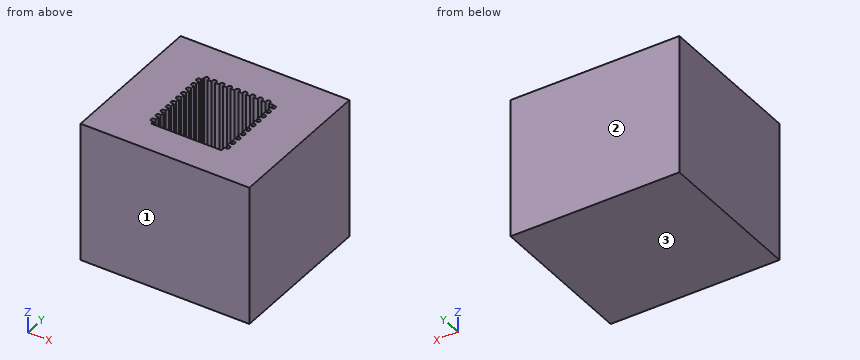
```python
from build123d import *

# Parameters (mm, degrees)
SKETCH1_W           = 504
SKETCH1_H           = 454
BOSS_EXTRUDE1_DEPTH = 416
SKETCH2_W           = 260
SKETCH2_H           = 260
CUT_EXTRUDE1_DEPTH  = 260
BOSS_EXTRUDE2_DEPTH = 260
SKETCH6_R           = 6.5
CUT_EXTRUDE2_DEPTH  = 260
LPATTERN3_COUNT     = 10
LPATTERN3_PITCH     = 23
SKETCH7_R           = 6.5
CUT_EXTRUDE3_DEPTH  = 260
LPATTERN4_COUNT     = 10
LPATTERN4_PITCH     = 23
SKETCH8_R           = 6.5
CUT_EXTRUDE4_DEPTH  = 260
LPATTERN5_COUNT     = 9
LPATTERN5_PITCH     = 23


with BuildPart() as part:
    # Sketch1 → Boss-Extrude1 (new body)
    with BuildSketch(Plane.XY):
        Rectangle(SKETCH1_W, SKETCH1_H)
    extrude(amount=-BOSS_EXTRUDE1_DEPTH)

    # Sketch2 → Cut-Extrude1 (cut)
    with BuildSketch(Plane.XY):
        Rectangle(SKETCH2_W, SKETCH2_H)
    extrude(amount=-CUT_EXTRUDE1_DEPTH, mode=Mode.SUBTRACT)

    # Sketch5 → Boss-Extrude2 (add)
    with BuildSketch(Plane.XY):
        Polygon((-105, 130), (-130, 130), (-130, 105), (-130, -130), (-105, -130), (-105, 105), (105, 105), (105, -130), (130, -130), (130, 105), (130, 130), (105, 130), align=None)
    extrude(amount=-BOSS_EXTRUDE2_DEPTH)

    # Sketch6 → Cut-Extrude2 (cut)
    with BuildSketch(Plane.XY):
        with Locations((-109.593002072, 92.497724269)):
            Circle(SKETCH6_R)
    cut_extrude2 = extrude(amount=-CUT_EXTRUDE2_DEPTH, mode=Mode.SUBTRACT)

    # LPattern3: Cut-Extrude2 ×10
    with Locations(*[(0, -i * LPATTERN3_PITCH, 0) for i in range(1, LPATTERN3_COUNT)]):
        add(cut_extrude2, mode=Mode.SUBTRACT)

    # Sketch7 → Cut-Extrude3 (cut)
    with BuildSketch(Plane.XY):
        with Locations((110.371561269, 97.109609101)):
            Circle(SKETCH7_R)
    cut_extrude3 = extrude(amount=-CUT_EXTRUDE3_DEPTH, mode=Mode.SUBTRACT)

    # LPattern4: Cut-Extrude3 ×10
    with Locations(*[(0, -i * LPATTERN4_PITCH, 0) for i in range(1, LPATTERN4_COUNT)]):
        add(cut_extrude3, mode=Mode.SUBTRACT)

    # Sketch8 → Cut-Extrude4 (cut)
    with BuildSketch(Plane.XY):
        with Locations((-96.786646696, 108.681954404)):
            Circle(SKETCH8_R)
    cut_extrude4 = extrude(amount=-CUT_EXTRUDE4_DEPTH, mode=Mode.SUBTRACT)

    # LPattern5: Cut-Extrude4 ×9
    with Locations(*[(i * LPATTERN5_PITCH, 0, 0) for i in range(1, LPATTERN5_COUNT)]):
        add(cut_extrude4, mode=Mode.SUBTRACT)


solid = part.part
```
Verification items for the finished model (mm, model axes). Face numbers are marked on the shaded views. Round coordinates to 2 decimals unless told otherwise and drop trailing zeros. Use CSV: the item, a comma, the result in double quotes.
(1) Thickness scan on probe 1 along Y at (x, z) = (-42.5, -87); probe 2 along X at (y, z) = (9.5, -227); probe 3 along Z at (x, y) = (59, 16). Record the ranges inside material, lowest first. Write a range as from..to.
Entries:
probe 1,"-227..-130, 105..227"
probe 2,"-252..-105, 105..105.58, 115.16..252"
probe 3,"-416..-260"
(2) Gauge pin test, flat end, axial feed: pin 1 Ø10.5 at (x, y) = (18.21, 108.68) entering from +Z. Record the tip position at first contact, or that the pin passes through.
Entries:
pin 1,"z = -260"
(3) Mould release check, pull along Y, two halves, no side actions. Record for the marked faces 1, 2 and 3: released by +Y, released by -Y, zero draft, split by the parting line, or undercut.
Entries:
face 1,"released by -Y"
face 2,"released by +Y"
face 3,"zero draft"
